```python
from build123d import *

# Parameters (mm, degrees)
SKETCH1_R                                       = 51.5
BOSS_EXTRUDE1_DEPTH                             = 10
CSK_FOR_M5_FLAT_HEAD_MACHINE_SCREW1_D           = 5.5
CSK_FOR_M5_FLAT_HEAD_MACHINE_SCREW1_CSINK_D     = 10.4
CSK_FOR_M5_FLAT_HEAD_MACHINE_SCREW1_CSINK_ANGLE = 90
CIRPATTERN1_COUNT                               = 8
F_1_5_1_5_DIAMETER_HOLE9_D                      = 1.5
F_1_5_1_5_DIAMETER_HOLE4_D                      = 1.5
F_1_5_1_5_DIAMETER_HOLE5_D                      = 1.5
F_1_5_1_5_DIAMETER_HOLE8_D                      = 1.5
CIRPATTERN2_COUNT                               = 20
CIRPATTERN3_COUNT                               = 14
CIRPATTERN7_COUNT                               = 6
CIRPATTERN8_COUNT                               = 4


with BuildPart() as part:
    # Sketch1 → Boss-Extrude1 (new body)
    with BuildSketch(Plane(origin=(0, 0, 0), x_dir=(1, 0, 0), z_dir=(0, 1, 0))):
        with Locations(Location((0, 0, 0), (0, 0, 270))):
            Circle(SKETCH1_R)
    extrude(amount=-BOSS_EXTRUDE1_DEPTH)

    # CSK for M5 Flat Head Machine Screw1 (through all)
    with Locations(Plane(origin=(0, 0, 0), x_dir=(1, 0, 0), z_dir=(0, 1, 0))):
        with Locations((0, 45)):
            csk_for_m5_flat_head_machine_screw1 = CounterSinkHole(CSK_FOR_M5_FLAT_HEAD_MACHINE_SCREW1_D / 2, CSK_FOR_M5_FLAT_HEAD_MACHINE_SCREW1_CSINK_D / 2, counter_sink_angle=CSK_FOR_M5_FLAT_HEAD_MACHINE_SCREW1_CSINK_ANGLE)

    # CirPattern1: CSK for M5 Flat Head Machine Screw1 ×8 about axis
    cirpattern1_axis = Axis((0, 0, 0), (0, 1, 0))
    for i in range(1, CIRPATTERN1_COUNT):
        add(csk_for_m5_flat_head_machine_screw1.rotate(cirpattern1_axis, i * 360 / CIRPATTERN1_COUNT), mode=Mode.SUBTRACT)

    # 1.5 _1.5_ Diameter Hole9 (through all)
    with Locations(Plane(origin=(0, -10, 0), x_dir=(-1, 0, 0), z_dir=(0, -1, 0))):
        with Locations((0, 5)):
            f_1_5_1_5_diameter_hole9 = Hole(F_1_5_1_5_DIAMETER_HOLE9_D / 2)

    # 1.5 _1.5_ Diameter Hole4 (through all)
    with Locations(Plane(origin=(0, 0, 0), x_dir=(1, 0, 0), z_dir=(0, 1, 0))):
        with Locations((0, 20)):
            f_1_5_1_5_diameter_hole4 = Hole(F_1_5_1_5_DIAMETER_HOLE4_D / 2)

    # 1.5 _1.5_ Diameter Hole5 (through all)
    with Locations(Plane(origin=(0, 0, 0), x_dir=(1, 0, 0), z_dir=(0, 1, 0))):
        with Locations((0, 30)):
            f_1_5_1_5_diameter_hole5 = Hole(F_1_5_1_5_DIAMETER_HOLE5_D / 2)

    # 1.5 _1.5_ Diameter Hole8 (through all)
    with Locations(Plane(origin=(0, 0, 0), x_dir=(1, 0, 0), z_dir=(0, 1, 0))):
        with Locations((0, 12.5)):
            f_1_5_1_5_diameter_hole8 = Hole(F_1_5_1_5_DIAMETER_HOLE8_D / 2)

    # CirPattern2: 1.5 _1.5_ Diameter Hole5 ×20 about axis
    cirpattern2_axis = Axis((0, 0, 0), (0, 1, 0))
    for i in range(1, CIRPATTERN2_COUNT):
        add(f_1_5_1_5_diameter_hole5.rotate(cirpattern2_axis, i * 360 / CIRPATTERN2_COUNT), mode=Mode.SUBTRACT)

    # CirPattern3: 1.5 _1.5_ Diameter Hole4 ×14 about axis
    cirpattern3_axis = Axis((0, 0, 0), (0, 1, 0))
    for i in range(1, CIRPATTERN3_COUNT):
        add(f_1_5_1_5_diameter_hole4.rotate(cirpattern3_axis, i * 360 / CIRPATTERN3_COUNT), mode=Mode.SUBTRACT)

    # CirPattern7: 1.5 _1.5_ Diameter Hole8 ×6 about axis
    cirpattern7_axis = Axis((0, 0, 0), (0, 1, 0))
    for i in range(1, CIRPATTERN7_COUNT):
        add(f_1_5_1_5_diameter_hole8.rotate(cirpattern7_axis, i * 360 / CIRPATTERN7_COUNT), mode=Mode.SUBTRACT)

    # CirPattern8: 1.5 _1.5_ Diameter Hole9 ×4 about axis
    cirpattern8_axis = Axis((0, 0, 0), (0, 1, 0))
    for i in range(1, CIRPATTERN8_COUNT):
        add(f_1_5_1_5_diameter_hole9.rotate(cirpattern8_axis, i * 360 / CIRPATTERN8_COUNT), mode=Mode.SUBTRACT)


solid = part.part
```
Here's how the part is built. I have some questions about the finished solid (model axes, mm). Give positions to 0.01 mm unless a question says otherwise; leave off trailing zeros. Write each loop counter-clockwise with the first axis right and the second up, starting at its lowest first coordinate (ties: lowest second). Pieces come first, ordered by that corner, then holes. Notation, with made-up numbers: M 87,20 L 100,20 A24 ccw 100,38 Z; hole C 2,51 d8. An arc over 180 degrees is marked long. Put each result on its own line as item: value. Start each with the question number.
Item 1: Will these pins go through, and if not, where does the flat tip stop? pin 1 (2 mm diameter, centred on x = 0, z = -5, fed in from +Y); pin 2 (5 mm diameter, centred on x = -28.5, y = -7.5, fed in from +Z); pin 3 (3 mm diameter, centred on x = -38.5, y = -2.5, fed in from -Z); pin 4 (6 mm diameter, centred on y = -6, z = -9, fed in from -X).
Item 2: If we section it at B-B, the plane z = -45: Write out the boundary of the cut face in (x, y).
Item 3: I need wall thicknesses on L1, parallel to Z at x = 18, y = -7.5; L2, parallel to Z at x = 29, y = -6.75; L3, parallel to X at y = -6.75, z = 29.5. Which ranges of each line are inside material? Lowest first, please. Write a range as from..to.
Item 4: If we section it at C-C, the plane y = -7: Count the separate pieces of the cut face and the enclosed holes in it, then the cut area to 3 significant figures.
Item 5: Thinking about a two-plate mould opening in Z: for faces 1 (the conical face through (31.7, -2.33, 34.69)), 2 (the flat face through (1, -10, -1)), 3 (the cylindrical face through (-45.69, -4.93, 23.76)), 4 (the cylindrical face through (0.358, -6.278, -47.727)), which applies, +Z half, -Z half, draft (parallel to the pull), parting line (faces both ways), or undercut?
Item 6: If we section it at A-A, the plane x = -45: Write out the boundary of the cut face in (y, z).
Values:
1. pin 1: y = 0
1. pin 2: z = 44.46
1. pin 3: z = -35.82
1. pin 4: x = -51.15
2. outline: M -25.04,-10 L -2.75,-10 L -2.75,-2.45 L -5.2,0 L -25.04,0 Z; M 2.75,-10 L 25.04,-10 L 25.04,0 L 5.2,0 L 2.75,-2.45 Z
3. L1: -48.25..-24.92, -23.62..23.62, 24.92..48.25
3. L2: -42.56..-9.86, -8.68..8.68, 9.86..42.56
3. L3: -42.21..-33.3, -30.34..-0.56, 0.56..30.34, 33.3..42.21
4. separate pieces: 1
4. enclosed holes: 52
4. area: 8,060 mm²
5. face 1: undercut
5. face 2: draft
5. face 3: parting line
5. face 4: undercut
6. outline: M -10,-25.04 L 0,-25.04 L 0,-5.2 L -2.45,-2.75 L -10,-2.75 Z; M -10,2.75 L -2.45,2.75 L 0,5.2 L 0,25.04 L -10,25.04 Z
